from build123d import *

# Parameters (mm, degrees)
SKETCH1_R           = 2.5
SKETCH1_R_2         = 6
BOSS_EXTRUDE1_DEPTH = 10


with BuildPart() as part:
    # Sketch1 → Boss-Extrude1 (new body)
    with BuildSketch(Plane.XY):
        with BuildLine():
            Line((-52, 55), (52, 55))
            ThreePointArc((52, 55), (54.121320344, 54.121320344), (55, 52))
            Line((55, 52), (55, -52))
            ThreePointArc((55, -52), (54.121320344, -54.121320344), (52, -55))
            Line((52, -55), (-52, -55))
            ThreePointArc((-52, -55), (-54.121320344, -54.121320344), (-55, -52))
            Line((-55, -52), (-55, 52))
            ThreePointArc((-55, 52), (-54.121320344, 54.121320344), (-52, 55))
        make_face()
        with Locations((47, 47)):
            Circle(SKETCH1_R, mode=Mode.SUBTRACT)
        with Locations(Location((47, -47, 0), (0, 0, 180))):
            Circle(SKETCH1_R, mode=Mode.SUBTRACT)
        with Locations((-47, -47)):
            Circle(SKETCH1_R, mode=Mode.SUBTRACT)
        with Locations(Location((-47, 47, 0), (0, 0, 180))):
            Circle(SKETCH1_R, mode=Mode.SUBTRACT)
        with Locations((0, 37)):
            Circle(SKETCH1_R_2, mode=Mode.SUBTRACT)
    extrude(amount=BOSS_EXTRUDE1_DEPTH)


solid = part.part
Design review of the part built by this model. Coordinates are the model's own, in mm. Coordinates: 2 decimals unless noted, no trailing zeros. Write each loop counter-clockwise with the first axis right and the second up, starting at its lowest first coordinate (ties: lowest second). Pieces come first, ordered by that corner, then holes. Notation, with made-up numbers: (-8, 41.5) -> (-3, 41.5) arc R28 cw to (-3, 61.5) -> close; hole circle Ø10 at (12.5, -2.75). An arc over 180 degrees is marked (long way). Write each question's results on one line, items separated by ' | '. Start each with the question number.
(1) Take a section at A-A on y = 37. Write out the cut boundary in (x, z), and give its area (3 significant figures).
(2) The part is to be moulded in two halves that separate along X. For faces 1 (the face through (44.69, -46.04, 4.93)), 2 (the face through (49.31, 46.04, 4.93)), 3 (the face through (55, 1, 5)), 4 (the face through (-54.14, 54.1, 4.93)), say which applies: pulls with the +X half, pulls with the -X half, needs draft (parallel to the pull), parting line crosses it, or undercut.
(3) For line 1 along Y through (x, z) = (47, 7.5); line 2 along Y through (x, z) = (0, 6.25), list the stretches that pass through material, from the lowest coordinate up. Write a range as from..to.
(4) Take a section at B-B on x = 47. Write out the cut boundary in (y, z).
(5) Clearance check with a flat-ended pin moving along its axis: P1, Ø7, axis at x = 0, y = 37, coming from the -Z side. State where the tip first meets the part, or that it passes through.
(6) Take a section at C-C on z = 5.5. Write out the cut boundary in (x, y), and give its area (3 significant figures).
(7) Take a section at D-D on x = 1.5. Write out the cut boundary in (y, z), and give its area (3 significant figures).
Results found:
1) outline: (-55, 0) -> (-6, 0) -> (-6, 10) -> (-55, 10) -> close; (6, 0) -> (55, 0) -> (55, 10) -> (6, 10) -> close | area: 980 mm2
2) face 1: undercut | face 2: undercut | face 3: pulls with the +X half | face 4: pulls with the -X half
3) line 1: y = -55..-49.5, -44.5..44.5, 49.5..55 | line 2: y = -55..31, 43..55
4) outline: (-55, 0) -> (-49.5, 0) -> (-49.5, 10) -> (-55, 10) -> close; (-44.5, 0) -> (44.5, 0) -> (44.5, 10) -> (-44.5, 10) -> close; (49.5, 0) -> (55, 0) -> (55, 10) -> (49.5, 10) -> close
5) P1: passes through
6) outline: (-55, -52) arc R3 ccw to (-52, -55) -> (52, -55) arc R3 ccw to (55, -52) -> (55, 52) arc R3 ccw to (52, 55) -> (-52, 55) arc R3 ccw to (-55, 52) -> close; hole circle Ø5 at (-47, -47); hole circle Ø5 at (-47, 47); hole circle Ø12 at (0, 37); hole circle Ø5 at (47, -47); hole circle Ø5 at (47, 47) | area: 11,900 mm2
7) outline: (-55, 0) -> (31.19, 0) -> (31.19, 10) -> (-55, 10) -> close; (42.81, 0) -> (55, 0) -> (55, 10) -> (42.81, 10) -> close | area: 984 mm2
